Design review of the part built by this model. Coordinates are the model's own, in mm. Coordinates: 2 decimals unless noted, no trailing zeros. Write each loop counter-clockwise with the first axis right and the second up, starting at its lowest first coordinate (ties: lowest second). Pieces come first, ordered by that corner, then holes. Notation, with made-up numbers: (46, 18) -> (68, 18) arc R12 cw to (68, 35) -> close; hole circle Ø4 at (79, 72.5). An arc over 180 degrees is marked (long way). One line per question, with ' | ' between items. Start each with the question number.
Q1. Add section C-C on y = -2.15. State the section outline as (x, z) points, and give its area (3 significant figures).
Q2. Add section D-D on x = 275. State the section outline as (y, z) points.
Q3. Add section B-B on x = 156. State the section outline as (y, z) points, and give its area (3 significant figures).
Q4. Wall thickness on probe 1 along X at (y, z) = (-5.05, -348); probe 2 along Z at (x, y) = (189.5, -4.25); probe 3 along X at (y, z) = (-2.9, -387): over which ranges is each line inside the solid? List them lowest first.
Q5. For P1, Ø3, axis at y = -4, z = -130.5, coming from the +X side; P2, Ø1, axis at y = -1, z = -204.5, coming from the +X side; P3, Ø2, axis at y = -2, z = -62, coming from the +X side, all flat-tipped, find the tip position at first contact; note any pin that passes through.
Q6. Add section A-A on z = -345.5. State the section outline as (x, y) points.
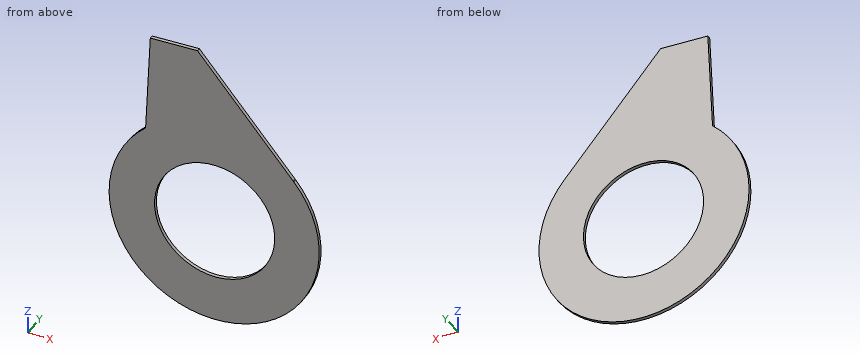
from build123d import *

# Parameters (mm, degrees)
F0_R     = 100
F1_DEPTH = 6


with BuildPart() as f1:
    # F0 (on Front) → F1 (new body)
    with BuildSketch(Plane.XZ):
        with BuildLine():
            Line((262.411714, -184.528433), (263.519588, -185.804495))
            ThreePointArc((263.519588, -185.804495), (262.967193, -185.165125), (262.411714, -184.528433))
        make_face()
        with BuildLine():
            Line((24.723456, -3.519507), (16.907266, -167.289172))
            ThreePointArc((16.907266, -167.289172), (117.873865, -474.095573), (263.519588, -185.804495))
            Line((263.519588, -185.804495), (262.411714, -184.528433))
            Line((262.411714, -184.528433), (103.280142, -1.238735))
            Line((103.280142, -1.238735), (24.723456, -3.519507))
        make_face()
        with Locations((131.77757, -297.979613)):
            Circle(F0_R, mode=Mode.SUBTRACT)
    extrude(amount=F1_DEPTH)


solid = f1.part
Output values:
1) outline: (16.91, -167.29) arc R174.81 ccw (long way) to (263.52, -185.8) arc R174.79 ccw to (262.41, -184.53) -> (103.28, -1.24) -> (24.72, -3.52) -> close; hole circle Ø200 at (131.78, -297.98) | area: 83,600 mm2
2) outline: (-6, -398.83) -> (0, -398.83) -> (0, -200.71) -> (-6, -200.71) -> close
3) outline: (-6, -472.78) -> (0, -472.78) -> (0, -395) -> (-6, -395) -> close; (-6, -200.96) -> (0, -200.96) -> (0, -61.96) -> (-6, -61.96) -> close | area: 1,300 mm2
4) probe 1: x = -37.07 to 45.19, 218.37 to 298.99 | probe 2: z = -464.49 to -379.64, -216.32 to -100.55 | probe 3: x = -20.54 to 86.22, 177.33 to 282.46
5) P1: stops at x = 216.81 | P2: stops at x = 277.86 | P3: stops at x = 156.9
6) outline: (-37.77, -6) -> (43.79, -6) -> (43.79, 0) -> (-37.77, 0) -> close; (219.77, -6) -> (299.69, -6) -> (299.69, 0) -> (219.77, 0) -> close
